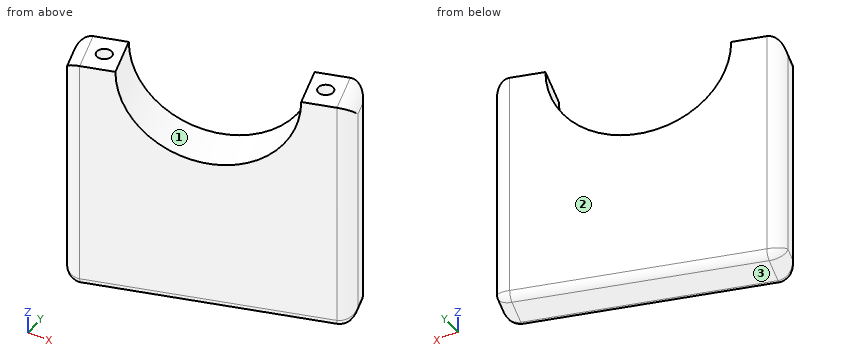
from build123d import *

# Parameters (mm, degrees)
PAD005_DEPTH      = 31
PAD005_DEPTH_BACK = 1
SKETCH022_R       = 11.2
POCKET006_DEPTH   = 15.7868758107
FILLET001_R       = 2
FILLET002_R       = 2
FILLET003_R       = 1
SKETCH026_R       = 1
SKETCH026_R_2     = 1.795314
SKETCH026_R_3     = 4.028245
POCKET008_DEPTH   = 12


with BuildPart() as part:
    # Sketch017 → Pad005 (new body, two sides)
    with BuildSketch(Plane.XY) as pad005_sk:
        Polygon((-6.1017054199, 68.7296820229), (-39.5723718786, 58.4966723576), (-37.8181416502, 52.7588438218), (-4.3474751915, 62.9918534871), align=None)
    extrude(amount=PAD005_DEPTH)
    extrude(pad005_sk.sketch, amount=-PAD005_DEPTH_BACK)

    # Sketch022 → Pocket006 (cut, through all)
    with BuildSketch(Plane(origin=(-19.7381564076, 64.5606005697, 0), x_dir=(-0.956304756, -0.2923717047, 0), z_dir=(-0.2923717047, 0.956304756, 0))):
        with Locations((3.2404756144, 31)):
            Circle(SKETCH022_R)
    extrude(amount=-POCKET006_DEPTH, mode=Mode.SUBTRACT)

    # Fillet001
    fillet001_edges = [part.edges().sort_by_distance(p)[0] for p in [
        (-39.572372, 58.496672, 15),
        (-37.818142, 52.758844, 15),
        (-38.695257, 55.627758, -1),
        (-38.695257, 55.627758, 31),
    ]]
    fillet(fillet001_edges, radius=FILLET001_R)

    # Fillet002
    fillet002_edges = [part.edges().sort_by_distance(p)[0] for p in [
        (-4.347475, 62.991853, 15),
        (-6.101705, 68.729682, 15),
        (-5.22459, 65.860768, -1),
        (-5.22459, 65.860768, 31),
    ]]
    fillet(fillet002_edges, radius=FILLET002_R)

    # Fillet003
    fillet003_edges = [part.edges().sort_by_distance(p)[0] for p in [
        (-22.837039, 63.613177, -1),
        (-21.082808, 57.875349, -1),
    ]]
    fillet(fillet003_edges, radius=FILLET003_R)

    # Sketch026 → Pocket008 (cut)
    with BuildSketch(Plane.XY.offset(31)):
        with Locations((-9.1932550429, 64.6474251804)):
            Circle(SKETCH026_R)
        with Locations((-34.7265920272, 56.8411006643)):
            Circle(SKETCH026_R)
        with Locations((66.962929, 24.575243)):
            Circle(SKETCH026_R_2)
        with Locations((61.462162, -12.93002)):
            Circle(SKETCH026_R_3)
    extrude(amount=-POCKET008_DEPTH, mode=Mode.SUBTRACT)


solid = part.part
The listing builds one solid part. Answer for the finished solid, in the listing's coordinates (mm). Face numbers are marked on the shaded views. Round coordinates to 2 decimals unless told otherwise and drop trailing zeros. Order: outer loops, then holes, each group sorted by start corner. A loop starts at its lowest first (then second) coordinate and runs counter-clockwise, first axis right, second up. Notation, with made-up numbers: (2, 60) -> (8, 60) arc R17 ccw to (8, 87) -> close; hole circle Ø2 at (76.25, 76.25). An arc over 180 degrees is marked (long way). One line per item, written item: value.
Item 1: Given P1, Ø12, axis at x = -13, z = 24.5, coming from the -Y side; P2, Ø1, axis at x = -12.5, z = 18.5, coming from the +Y side; P3, Ø4, axis at x = -14, z = 5.5, coming from the -Y side, each flat-ended and moving along its own axis, determine where each tip first touches the part or whether it passes through.
Taken from the geometry:
P1: stops at y = 58.99
P2: stops at y = 66.93
P3: stops at y = 59.43
Item 2: Find section A-A, the plane z = 26. Give the vertices of the cut face in (x, y).
Taken from the geometry:
outline: (-38.99, 56.58) -> (-38.4, 54.67) arc R2 ccw to (-35.91, 53.34) -> (-30.67, 54.95) -> (-32.42, 60.68) -> (-37.66, 59.08) arc R2 ccw to start; (-13.25, 66.54) -> (-11.5, 60.81) -> (-6.26, 62.41) arc R2 ccw to (-4.93, 64.9) -> (-5.52, 66.82) arc R2 ccw to (-8.01, 68.14) -> close; hole circle Ø2 at (-34.73, 56.84); hole circle Ø2 at (-9.19, 64.65)
Item 3: Find section B-B, the plane z = 12.5. Give the vertices of the cut face in (x, y), then the cut area to 3 significant figures.
Taken from the geometry:
outline: (-38.99, 56.58) -> (-38.4, 54.67) arc R2 ccw to (-35.91, 53.34) -> (-6.26, 62.41) arc R2 ccw to (-4.93, 64.9) -> (-5.52, 66.82) arc R2 ccw to (-8.01, 68.14) -> (-37.66, 59.08) arc R2 ccw to start
area: 207 mm2
Item 4: Straight lines are drawn through the part: L1, parallel to Y at x = -30, z = 20.5; L2, parallel to X at y = 64, z = 25.5; L3, parallel to Z at x = -14, y = 61.75. For each, find the intervals that lie inside material, in ascending order.
Taken from the geometry:
L1: y = 55.15 to 61.42
L2: x = -12.75 to -9.96, -8.43 to -4.87
L3: z = -1 to 23.07
Item 5: Find section C-C, the plane z = 20.5. Give the vertices of the cut face in (x, y).
Taken from the geometry:
outline: (-38.99, 56.58) -> (-38.4, 54.67) arc R2 ccw to (-35.91, 53.34) -> (-24.81, 56.74) -> (-26.56, 62.47) -> (-37.66, 59.08) arc R2 ccw to start; (-19.11, 64.75) -> (-17.36, 59.01) -> (-6.26, 62.41) arc R2 ccw to (-4.93, 64.9) -> (-5.52, 66.82) arc R2 ccw to (-8.01, 68.14) -> close; hole circle Ø2 at (-34.73, 56.84); hole circle Ø2 at (-9.19, 64.65)
Item 6: For a pull along X with two mould halves and no side action, classify the marked faces 1, 2 and 3 as released by +X, released by -X, zero draft, split by the parting line, or undercut.
Taken from the geometry:
face 1: undercut
face 2: released by -X
face 3: zero draft
